Can you work these out from the drawing? Everything is in mm from the part's minimum corner. A direction names the side the tool comes from. Coordinates: 2 decimals unless noted, no trailing zeros. Loops run counter-clockwise (first coordinate to the right, second up) from the corner with the lowest first, then second, coordinate; pieces in that order, holes last. Notation, with made-up numbers: (62.25, 64.25) -> (115.25, 64.25) arc R10 ccw to (115.25, 71.25) -> close; hole circle Ø2 at (59, 34.25). An arc over 180 degrees is marked (long way). Use one line per item in the form item = value. Start each with the question number.
(1) On a 3-axis mill with a long thin cutter (end or side, diameter ignored), from which of +Z, -Z, +X, -X, +Y, -Y can I reach the whole of each face in a straight line? I mean the marked faces 1 and 2. Say none if no direction works.
(2) Imagine slicing it at C-C (z = 26). List the corners of the cut face in (x, y) for me, plus the area to 3 significant figures.
(3) Imagine slicing it at B-B (y = 11.75). List the corners of the cut face in (x, z) for me.
(4) I'm going to push flat-ended pins straight in: pin 1 (1 mm diameter, centred on y = 3, z = 11, fed in from -X); pin 2 (3 mm diameter, centred on x = 5.5, z = 15, fed in from +Y); pin 3 (1.6 mm diameter, centred on x = 4, y = 11.5, fed in from +Z). Where does each tip first touch, or does it pass through?
(5) Imagine slicing it at A-A (z = 17.5). List the corners of the cut face in (x, y) for me.
(6) I need wall thicknesses on line 1 (Y direction, x = 5, z = 19.75); line 2 (Y direction, x = 1, z = 10); line 3 (Y direction, x = 1, z = 26.5). Which ranges of each line are inside material? Lowest first, please. Write a range as [from, to].
(7) Imagine slicing it at D-D (y = 2.5). List the corners of the cut face in (x, z) for me, plus the area to 3 significant figures.
(8) Thinking about a two-plate mould opening in Z: for the marked faces 3, 4 and 5, which applies, released by +Z, released by -Z, zero draft, split by the parting line, or undercut?
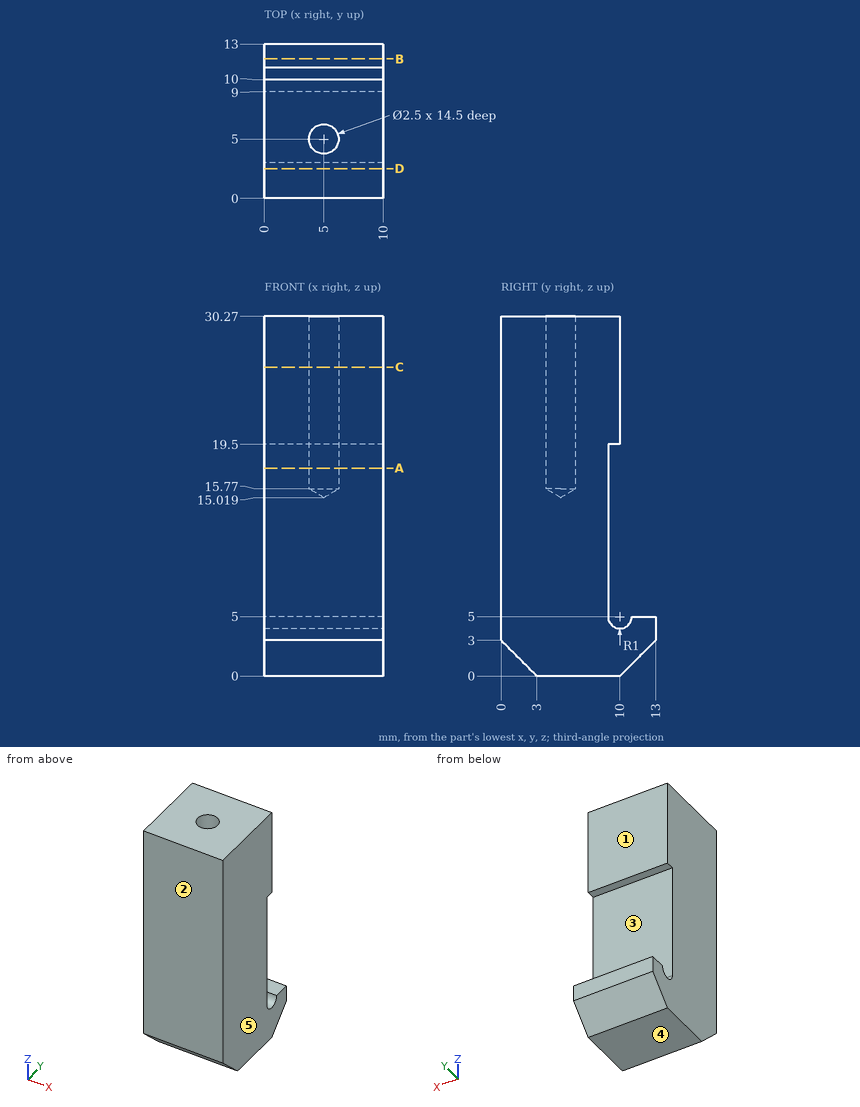
Worked out:
q1.face_1 = +Z, +X, -X, +Y
q1.face_2 = +Z, -Z, +X, -X, -Y
q2.outline = (0, 0) -> (10, 0) -> (10, 10) -> (0, 10) -> close; hole circle Ø2.5 at (5, 5)
q2.area = 95.1 mm2
q3.outline = (0, 1.75) -> (10, 1.75) -> (10, 5) -> (0, 5) -> close
q4.pin_1 = 0
q4.pin_2 = 9
q4.pin_3 = 5
q5.outline = (0, 0) -> (10, 0) -> (10, 9) -> (0, 9) -> close; hole circle Ø2.5 at (5, 5)
q6.line_1 = [0, 3.75], [6.25, 10]
q6.line_2 = [0, 9]
q6.line_3 = [0, 10]
q7.outline = (0, 0.5) -> (10, 0.5) -> (10, 30.27) -> (0, 30.27) -> close
q7.area = 298 mm2
q8.face_3 = undercut
q8.face_4 = released by -Z
q8.face_5 = zero draft
